For this review, take the finished solid that the model builds, in its own axes (mm). A direction names the side the tool comes from. Give positions to 0.01 mm unless a question says otherwise; leave off trailing zeros. Order: outer loops, then holes, each group sorted by start corner. A loop starts at its lowest first (then second) coordinate and runs counter-clockwise, first axis right, second up. Notation, with made-up numbers: (-28.5, 37) -> (-7.5, 37) arc R36 ccw to (-7.5, 76) -> close; hole circle Ø8 at (38.5, 50.25). An arc over 180 degrees is marked (long way). Return JSON: item names as keys, results as strings. Group by question number.
1) To check wall thickness, follow line 1 along X through (y, z) = (-0.9, -6.5); line 2 along X through (y, z) = (-1.2, -5.25); line 3 along Y through (x, z) = (13.5, -6). State the ranges of each line that lie inside material, in increasing order.
2) Add section C-C (x = 1.75). Give the boundary of the cut face in (y, z).
3) Add section B-B (z = -5.5). Give the boundary of the cut face in (x, y).
4) The part is to be moulded in two halves that separate along Z. For faces 3 (the face through (7, 0, -5)), 4 (the face through (3.2, -1, -7.5)), 5 (the face through (7.4, -1.2, 1.3)), 6 (the face through (7.4, -1.3, -9.2)), say which applies: released by +Z, released by -Z, zero draft, split by the parting line, or undercut.
5) Add section A-A (x = 11). Give the boundary of the cut face in (y, z).
6) Add section D-D (y = 0.75). Give the boundary of the cut face in (x, z).
7) Insertion check: P1, Ø3, axis at x = 7, z = -7.5, coming from the +Y side; P2, Ø1.5, axis at x = 8.5, y = 2, coming from the -Z side. Each pin has a flat end and moves straight along its axis. Give the tip position at first contact, or say it passes through.
8) For faces 1 (the face through (7, 1, 0)), 2 (the face through (14.4, -0.8, -9.1)), list the 3-axis set-ups (+Z, -Z, +X, -X, +Y, -Y) from which the entire face can be reached by the end or side of a thin tool; tool diameter is ignored.
from build123d import *

# Parameters (mm, degrees)
F1_DEPTH = 15
F3_D     = 3.4
F4_SIZE  = 1.5


with BuildPart() as f1:
    # F0 (on Right) → F1 (new body)
    with BuildSketch(Plane.YZ):
        Polygon((0, -10), (0, 0), (3, 0), (3, 2), (-2, 2), (-2, -10), align=None)
    extrude(amount=F1_DEPTH)

    # F3 (through all)
    with Locations(Plane.XZ.offset(2)):
        with Locations((4, -6), (11, -6)):
            Hole(F3_D / 2)

    # F4
    f4_edges = [f1.edges().sort_by_distance(p)[0] for p in [
        (0, 0.5, 2),
        (15, 0.5, 2),
        (0, -1, -10),
        (15, -1, -10),
        (7.5, -2, 2),
        (7.5, -2, -10),
    ]]
    chamfer(f4_edges, length=F4_SIZE)


solid = f1.part
Evaluation:
{
 "1": {"line 1": "0 to 2.38, 5.62 to 9.38, 12.62 to 15", "line 2": "0 to 2.47, 5.53 to 9.47, 12.53 to 15", "line 3": "-2 to 0"},
 "2": {"outline": "(-2, -8.5) -> (-0.5, -10) -> (0, -10) -> (0, 0) -> (3, 0) -> (3, 2) -> (-0.5, 2) -> (-2, 0.5) -> close"},
 "3": {"outline": "(0, -2) -> (2.38, -2) -> (2.38, 0) -> (0, 0) -> close; (5.62, -2) -> (9.38, -2) -> (9.38, 0) -> (5.62, 0) -> close; (12.62, -2) -> (15, -2) -> (15, 0) -> (12.62, 0) -> close"},
 "4": {"face 3": "zero draft", "face 4": "undercut", "face 5": "released by +Z", "face 6": "released by -Z"},
 "5": {"outline": "(-2, -8.5) -> (-0.5, -10) -> (0, -10) -> (0, -7.7) -> (-2, -7.7) -> close; (-2, -4.3) -> (0, -4.3) -> (0, 0) -> (3, 0) -> (3, 2) -> (-0.5, 2) -> (-2, 0.5) -> close"},
 "6": {"outline": "(0, 0) -> (15, 0) -> (15, 0.5) -> (13.5, 2) -> (1.5, 2) -> (0, 0.5) -> close"},
 "7": {"P1": "y = 0", "P2": "z = 0"},
 "8": {"face 1": "-Z, +X, -X, +Y", "face 2": "-Z, +X, +Y, -Y"}
}
